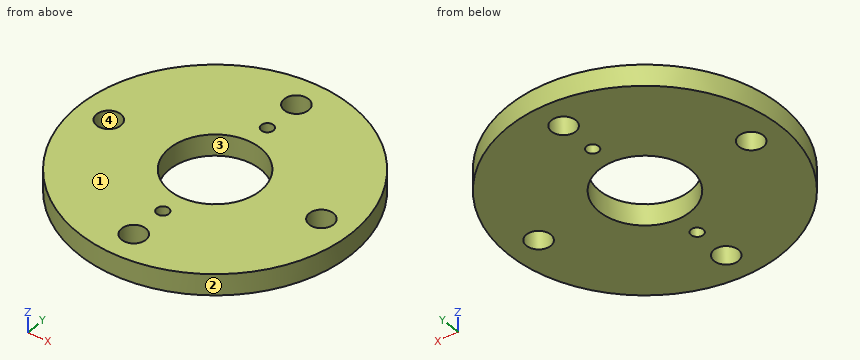
from build123d import *

# Parameters (mm, degrees)
CROQUIS1_R              = 45
SALIENTE_EXTRUIR1_DEPTH = 7
CROQUIS2_R              = 15
CORTAR_EXTRUIR1_DEPTH   = 8
CROQUIS3_R              = 4
CORTAR_EXTRUIR2_DEPTH   = 8
CROQUIS4_R              = 2
CORTAR_EXTRUIR3_DEPTH   = 8


with BuildPart() as part:
    # Croquis1 → Saliente-Extruir1 (new body)
    with BuildSketch(Plane.XY):
        Circle(CROQUIS1_R)
    extrude(amount=SALIENTE_EXTRUIR1_DEPTH)

    # Croquis2 → Cortar-Extruir1 (cut, through all)
    with BuildSketch(Plane.XY.offset(7)):
        Circle(CROQUIS2_R)
    extrude(amount=-CORTAR_EXTRUIR1_DEPTH, mode=Mode.SUBTRACT)

    # Croquis3 → Cortar-Extruir2 (cut, through all)
    with BuildSketch(Plane.XY.offset(7)):
        with Locations((0, 35)):
            Circle(CROQUIS3_R)
        with Locations((35, 0)):
            Circle(CROQUIS3_R)
        with Locations((0, -35)):
            Circle(CROQUIS3_R)
        with Locations((-35, 0)):
            Circle(CROQUIS3_R)
    extrude(amount=-CORTAR_EXTRUIR2_DEPTH, mode=Mode.SUBTRACT)

    # Croquis4 → Cortar-Extruir3 (cut, through all)
    with BuildSketch(Plane.XY.offset(7)):
        with Locations((0, 22.5)):
            Circle(CROQUIS4_R)
        with Locations((0, -22.5)):
            Circle(CROQUIS4_R)
    extrude(amount=-CORTAR_EXTRUIR3_DEPTH, mode=Mode.SUBTRACT)


solid = part.part
Input: part model. Units: mm. Frame: model coordinates. Face numbers are marked on the shaded views. Give positions to 0.01 mm unless a question says otherwise; leave off trailing zeros. Write each loop counter-clockwise with the first axis right and the second up, starting at its lowest first coordinate (ties: lowest second). Pieces come first, ordered by that corner, then holes.
Q1. First-contact query: P1, Ø4, axis at y = -11.5, z = 3, coming from the -X side; P2, Ø2, axis at x = -11.5, z = 6, coming from the -Y side; P3, Ø1.5, axis at x = -16, z = 4.5, coming from the +Y side; P4, Ø7, axis at x = 35, y = 0, coming from the -Z side. Flat tips, straight axial feed; report the tip coordinate or a pass-through.
Q2. Section D-D, the plane x = 11. Output: boundary loops of the cut face in (y, z), plus the area to 3 significant figures.
Q3. Pull-direction query (X, two-part tool) for the marked faces 1, 2, 3 and 4; classes: pulls with the +X half, pulls with the -X half, needs draft (parallel to the pull), parting line crosses it, or undercut.
Q4. Section C-C, the plane y = 22.5. Output: boundary loops of the cut face in (x, z), plus the area to 3 significant figures.
Q5. Section B-B, the plane z = 2.75. Output: boundary loops of the cut face in (x, y), plus the area to 3 significant figures.
Q6. Material intervals for probe 1 along Y at (x, z) = (0, 3.5); probe 2 along Y at (x, z) = (33.5, 5.5); probe 3 along X at (y, z) = (33, 1), sorted ascending.
Q7. Section A-A, the plane x = 0. Output: boundary loops of the cut face in (y, z), plus the area to 3 significant figures.
Filled in:
1. P1: stops at x = -43.99
1. P2: stops at y = -43.76
1. P3: stops at y = 42.34
1. P4: passes through
2. outline: (-43.63, 0) - (-10.2, 0) - (-10.2, 7) - (-43.63, 7) - close; (10.2, 0) - (43.63, 0) - (43.63, 7) - (10.2, 7) - close
2. area: 468 mm2
3. face 1: needs draft
3. face 2: parting line crosses it
3. face 3: undercut
3. face 4: undercut
4. outline: (-38.97, 0) - (-2, 0) - (-2, 7) - (-38.97, 7) - close; (2, 0) - (38.97, 0) - (38.97, 7) - (2, 7) - close
4. area: 518 mm2
5. outline: circle Ø90 at (0, 0); hole circle Ø8 at (-35, 0); hole circle Ø30 at (0, 0); hole circle Ø8 at (0, -35); hole circle Ø8 at (0, 35); hole circle Ø4 at (0, -22.5); hole circle Ø4 at (0, 22.5); hole circle Ø8 at (35, 0)
5. area: 5,430 mm2
6. probe 1: y = -45 to -39, -31 to -24.5, -20.5 to -15, 15 to 20.5, 24.5 to 31, 39 to 45
6. probe 2: y = -30.05 to -3.71, 3.71 to 30.05
6. probe 3: x = -30.59 to -3.46, 3.46 to 30.59
7. outline: (-45, 0) - (-39, 0) - (-39, 7) - (-45, 7) - close; (-31, 0) - (-24.5, 0) - (-24.5, 7) - (-31, 7) - close; (-20.5, 0) - (-15, 0) - (-15, 7) - (-20.5, 7) - close; (15, 0) - (20.5, 0) - (20.5, 7) - (15, 7) - close; (24.5, 0) - (31, 0) - (31, 7) - (24.5, 7) - close; (39, 0) - (45, 0) - (45, 7) - (39, 7) - close
7. area: 252 mm2
